Part model, mm, in its own coordinate system. A direction names the side the tool comes from. Round coordinates to 2 decimals unless told otherwise and drop trailing zeros. Loops run counter-clockwise (first coordinate to the right, second up) from the corner with the lowest first, then second, coordinate; pieces in that order, holes last.
from build123d import *

# Parameters (mm, degrees)
F1_DEPTH = 165.1
F3_DEPTH = 44.45


with BuildPart() as f1:
    # F0 (on Right) → F1 (new body)
    with BuildSketch(Plane.YZ):
        Polygon((-19.05, 0), (0, 0), (69.85, 0), (69.85, 31.75), (50.8, 31.75), (50.8, 44.45), (0, 44.45), (0, 31.75), (-19.05, 31.75), align=None)
    extrude(amount=F1_DEPTH)

    # F2 (on face) → F3 (cut, through all)
    with BuildSketch(Plane.XY.offset(44.45)):
        with BuildLine():
            Line((34.925, 25.4), (22.225, 25.4))
            ThreePointArc((22.225, 25.4), (34.925, 12.7), (47.625, 25.4))
            Line((47.625, 25.4), (34.925, 25.4))
        make_face()
        with BuildLine():
            ThreePointArc((142.875, 25.4), (130.175, 38.1), (117.475, 25.4))
            Line((117.475, 25.4), (130.175, 25.4))
            Line((130.175, 25.4), (142.875, 25.4))
        make_face()
        with BuildLine():
            Line((130.175, 25.4), (117.475, 25.4))
            ThreePointArc((117.475, 25.4), (130.175, 12.7), (142.875, 25.4))
            Line((142.875, 25.4), (130.175, 25.4))
        make_face()
        with BuildLine():
            ThreePointArc((47.625, 25.4), (34.925, 38.1), (22.225, 25.4))
            Line((22.225, 25.4), (34.925, 25.4))
            Line((34.925, 25.4), (47.625, 25.4))
        make_face()
    extrude(amount=-F3_DEPTH, mode=Mode.SUBTRACT)


solid = f1.part
1) Slice it at D-D, the plane x = 137. Give the cut face in (y, z).
Values:
outline: (-19.05, 0) - (14.69, 0) - (14.69, 44.45) - (0, 44.45) - (0, 31.75) - (-19.05, 31.75) - close; (36.11, 0) - (69.85, 0) - (69.85, 31.75) - (50.8, 31.75) - (50.8, 44.45) - (36.11, 44.45) - close
2) Mould opens along X. For faces 4 (the face through (81, 25, 0)), 5 (the face through (118.44, 30.26, 22.54)), 6 (the face through (0, 25, 18)), 7 (the face through (25.56, 33.98, 22.54)) say: released by +X, released by -X, zero draft, split by the parting line, or undercut.
Values:
face 4: zero draft
face 5: undercut
face 6: released by -X
face 7: undercut
3) Wall check: line 1 along X through (y, z) = (24.5, 6); line 2 along X through (y, z) = (25, 21); line 3 along Z through (x, y) = (77.5, -4.5). Give the ranges that are in metal, low to high.
Values:
line 1: x = 0 to 22.26, 47.59 to 117.51, 142.84 to 165.1
line 2: x = 0 to 22.23, 47.62 to 117.48, 142.87 to 165.1
line 3: z = 0 to 31.75
4) Drop flat-ended pins along their axis: pin 1 Ø23 at (x, y) = (130.175, 25.4) entering from +Z; pin 2 Ø5 at (x, z) = (139, 38.5) entering from +Y; pin 3 Ø6.5 at (x, z) = (112.5, 39) entering from -Y; pin 4 Ø15 at (x, y) = (117.5, 60) entering from +Z. Give the stop position or say it passes through.
Values:
pin 1: passes through
pin 2: stops at y = 50.8
pin 3: stops at y = 0
pin 4: stops at z = 31.75
5) Slice it at C-C, the plane z = 36. Give the cut face in (x, y) (3 decimals), then the cut area to 3 significant figures.
Values:
outline: (0, 0) - (165.1, 0) - (165.1, 50.8) - (0, 50.8) - close; hole circle Ø25.4 at (34.925, 25.4); hole circle Ø25.4 at (130.175, 25.4)
area: 7,370 mm2
6) Slice it at B-B, the plane x = 62. Give the cut face in (y, z).
Values:
outline: (-19.05, 0) - (69.85, 0) - (69.85, 31.75) - (50.8, 31.75) - (50.8, 44.45) - (0, 44.45) - (0, 31.75) - (-19.05, 31.75) - close
7) Slice it at A-A, the plane y = 25.4. Give the cut face in (x, z) (3 decimals), then the cut area to 3 significant figures.
Values:
outline: (0, 0) - (22.225, 0) - (22.225, 44.45) - (0, 44.45) - close; (47.625, 0) - (117.475, 0) - (117.475, 44.45) - (47.625, 44.45) - close; (142.875, 0) - (165.1, 0) - (165.1, 44.45) - (142.875, 44.45) - close
area: 5,080 mm2
8) Tool access for faces 1 (the face through (81, 26, 44.45)), 2 (the face through (81, 50.8, 38)), 3 (the face through (81, -9, 31.75)): list every direction of +Z, -Z, +X, -X, +Y, -Y with a clear straight run to the whole face (end or side of a thin tool).
Values:
face 1: +Z, +X, -X, +Y, -Y
face 2: +Z, +X, -X, +Y
face 3: +Z, +X, -X, -Y
